Work out the finished part from the listing and answer in its coordinate system (mm). Round coordinates to 2 decimals unless told otherwise and drop trailing zeros. Write each loop counter-clockwise with the first axis right and the second up, starting at its lowest first coordinate (ties: lowest second). Pieces come first, ordered by that corner, then holes. Notation, with made-up numbers: (29, 16) -> (79, 16) arc R20 ccw to (79, 27) -> close; hole circle Ø8 at (-9, 14). An arc over 180 degrees is marked (long way). One line per item, written item: value.
```python
from build123d import *

# Parameters (mm, degrees)
F1_R     = 3.175
F2_DEPTH = 3.175
F3_DEPTH = 3.175
F0_R     = 3.175
F4_DEPTH = 914.4
F5_W     = 25.4
F5_H     = 12.7
F5_R     = 3.175
F6_DEPTH = 3.175


with BuildPart() as f2:
    # F1 (on Right) → F2 (new body, symmetric)
    with BuildSketch(Plane.YZ):
        with BuildLine():
            ThreePointArc((-6.35, 6.35), (-12.7, 0), (-6.35, -6.35))
            ThreePointArc((-6.35, -6.35), (-1.8598719395, -4.4901280605), (0, 0))
            ThreePointArc((0, 0), (-1.8598719395, 4.4901280605), (-6.35, 6.35))
        make_face()
        with Locations((-6.35, 0)):
            Circle(F1_R, mode=Mode.SUBTRACT)
    extrude(amount=F2_DEPTH, both=True)

    # F1 (on Right) → F3 (join, symmetric)
    with BuildSketch(Plane.YZ):
        with BuildLine():
            Line((-6.35, -6.35), (6.35, -6.35))
            Line((6.35, -6.35), (6.35, 6.35))
            Line((6.35, 6.35), (-6.35, 6.35))
            ThreePointArc((-6.35, 6.35), (-1.8598719395, 4.4901280605), (0, 0))
            ThreePointArc((0, 0), (-1.8598719395, -4.4901280605), (-6.35, -6.35))
        make_face()
    extrude(amount=F3_DEPTH, both=True)

    # F0 (on Front) → F4 (join)
    with BuildSketch(Plane.XZ):
        Circle(F0_R)
    extrude(amount=-F4_DEPTH)

    # F5 (on Right) → F6 (join, symmetric)
    with BuildSketch(Plane.YZ):
        with Locations((914.4588708878, 0)):
            Rectangle(F5_W, F5_H)
        with Locations((923.234462738, 0)):
            Circle(F5_R, mode=Mode.SUBTRACT)
    extrude(amount=F6_DEPTH, both=True)


solid = f2.part
```
(1) Find section A-A on x = 0. Give the vertices of the cut face in (y, z) (3 decimals).
Reported:
outline: (-6.35, -6.35) -> (6.35, -6.35) -> (6.35, -3.175) -> (901.759, -3.175) -> (901.759, -6.35) -> (927.159, -6.35) -> (927.159, 6.35) -> (901.759, 6.35) -> (901.759, 3.175) -> (6.35, 3.175) -> (6.35, 6.35) -> (-6.35, 6.35) arc R6.35 ccw to start; hole circle Ø6.35 at (-6.35, 0); hole circle Ø6.35 at (923.234, 0)
(2) Consider probe 1 along Y at (x, z) = (-3, -5.5); probe 2 along Y at (x, z) = (-1, -1.25); probe 3 along X at (y, z) = (817.5, -1). Determine where each line is inside the solid, lowest interval first.
Reported:
probe 1: y = -9.52 to 6.35, 901.76 to 927.16
probe 2: y = -12.58 to -9.27, -3.43 to 920.32, 926.15 to 927.16
probe 3: x = -3.01 to 3.01
(3) Flat-ended cylindrical pins translate along their axes: pin 1 Ø1.5 at (y, z) = (139.5, -2.5) entering from +X; pin 2 Ø4 at (y, z) = (923.23, 0) entering from -X; pin 3 Ø1.5 at (x, y) = (1.5, 322.5) entering from +Z; pin 4 Ø3 at (x, z) = (1.5, -3.5) entering from -Y. Find the tip coordinate at first contact, or state that the pin passes through.
Reported:
pin 1: stops at x = 2.65
pin 2: passes through
pin 3: stops at z = 3.09
pin 4: stops at y = -12.38
(4) Find section B-B on y = 131. Give the vertices of the cut face in (x, z) (3 decimals), plus the area to 3 significant figures.
Reported:
outline: circle Ø6.35 at (0, 0)
area: 31.7 mm2
